```python
from build123d import *

# Parameters (mm, degrees)
CYLINDER084_R     = 2
CYLINDER084_DEPTH = 10
CYLINDER083_R     = 3.25
CYLINDER083_DEPTH = 10
CYLINDER082_R     = 2
CYLINDER082_DEPTH = 10
BOX069_W          = 8.5
BOX069_H          = 22
BOX069_DEPTH      = 25
BOX068_W          = 8
BOX068_H          = 22
BOX068_DEPTH      = 25


with BuildPart() as cylinder084:
    # Cylinder084 → Cylinder084 (new body)
    with BuildSketch(Plane(origin=(335, 287, 0), x_dir=(1, 0, 0), z_dir=(0, 0, 1))):
        Circle(CYLINDER084_R)
    extrude(amount=CYLINDER084_DEPTH)


with BuildPart() as cylinder083:
    # Cylinder083 → Cylinder083 (new body)
    with BuildSketch(Plane(origin=(335, 305, 17), x_dir=(1, 0, 0), z_dir=(0, -1, 0))):
        Circle(CYLINDER083_R)
    extrude(amount=CYLINDER083_DEPTH)


with BuildPart() as fusion049:
    # Cylinder082 → Cylinder082 (new body)
    with BuildSketch(Plane(origin=(335, 294, 0), x_dir=(1, 0, 0), z_dir=(0, 0, 1))):
        Circle(CYLINDER082_R)
    extrude(amount=CYLINDER082_DEPTH)

    # Fusion049: union Cylinder083
    add(cylinder083.part)


with BuildPart() as cube020:
    # Box069 → Box069 (new body)
    with BuildSketch(Plane(origin=(331, 278, 9), x_dir=(1, 0, 0), z_dir=(0, 0, 1))):
        with Locations((4.25, 11)):
            Rectangle(BOX069_W, BOX069_H)
    extrude(amount=BOX069_DEPTH)


with BuildPart() as antennaholder:
    # Box068 → Box068 (new body)
    with BuildSketch(Plane(origin=(331, 283, 0), x_dir=(1, 0, 0), z_dir=(0, 0, 1))):
        with Locations((4, 11)):
            Rectangle(BOX068_W, BOX068_H)
    extrude(amount=BOX068_DEPTH)

    # Cut061: cut Cube020
    add(cube020.part, mode=Mode.SUBTRACT)

    # Cut062: cut Fusion049
    add(fusion049.part, mode=Mode.SUBTRACT)

    # Cut063: cut Cylinder084
    add(cylinder084.part, mode=Mode.SUBTRACT)


solid = antennaholder.part
```
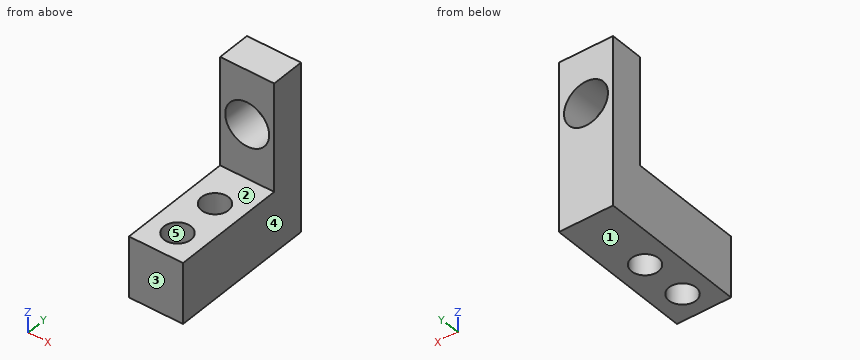
The listing builds one solid part. Answer for the finished solid, in the listing's coordinates (mm). Face numbers are marked on the shaded views. A direction names the side the tool comes from. Coordinates: 2 decimals unless noted, no trailing zeros. Loops run counter-clockwise (first coordinate to the right, second up) from the corner with the lowest first, then second, coordinate; pieces in that order, holes last. Notation, with made-up numbers: (-29, 2) - (-16, 2) arc R10 cw to (-16, 13) - close; hole circle Ø9 at (-15.5, 82). An arc over 180 degrees is marked (long way). Use a Markdown table: item, result. Add a question column.
1) The part is cut by section D-D, the plane x = 332.5. Give the vertices of the cut face in (y, z).
2) Given pin 1 (1 mm diameter, centred on x = 336.5, y = 287.5, fed in from +Z), flat-ended and moving along its own axis, determine where the tip first touches the part or whether it passes through.
3) The part is cut by section B-B, the plane x = 335. Give the vertices of the cut face in (y, z).
4) For the marked faces 1 and 2, determine the directions among +Z, -Z, +X, -X, +Y, -Y from which every point of the face is accessible in a straight line to the end or side of a thin tool.
5) The part is cut by section A-A, the plane y = 287. Give the vertices of the cut face in (x, z).
6) The mould has two halves that part along Y. Classify the marked faces 3, 4 and 5: released by +Y, released by -Y, zero draft, split by the parting line, or undercut.
7) Find the intervals of material crossed by line 1 (X direction, y = 303.35, z = 17); line 2 (Y direction, x = 333.5, z = 1); line 3 (Z direction, x = 335, y = 302.25), in increasing order.
8) The part is cut by section C-C, the plane y = 301.25. Give the vertices of the cut face in (x, z), and give its area (3 significant figures).
Here are the results:
| question | item | result |
|---|---|---|
| 1 | outline | (283, 0) - (305, 0) - (305, 14.92) - (300, 14.92) - (300, 9) - (283, 9) - close; (300, 19.08) - (305, 19.08) - (305, 25) - (300, 25) - close |
| 2 | pin 1 | stops at z = 9 |
| 3 | outline | (283, 0) - (285, 0) - (285, 9) - (283, 9) - close; (289, 0) - (292, 0) - (292, 9) - (289, 9) - close; (296, 0) - (305, 0) - (305, 13.75) - (300, 13.75) - (300, 9) - (296, 9) - close; (300, 20.25) - (305, 20.25) - (305, 25) - (300, 25) - close |
| 4 | face 1 | -Z, +X, -X, +Y, -Y |
| 4 | face 2 | +Z, +X, -X, -Y |
| 5 | outline | (331, 0) - (333, 0) - (333, 9) - (331, 9) - close; (337, 0) - (339, 0) - (339, 9) - (337, 9) - close |
| 6 | face 3 | released by -Y |
| 6 | face 4 | zero draft |
| 6 | face 5 | undercut |
| 7 | line 1 | x = 331 to 331.75, 338.25 to 339 |
| 7 | line 2 | y = 283 to 285.68, 288.32 to 292.68, 295.32 to 305 |
| 7 | line 3 | z = 0 to 13.75, 20.25 to 25 |
| 8 | outline | (331, 0) - (339, 0) - (339, 25) - (331, 25) - close; hole circle Ø6.5 at (335, 17) |
| 8 | area | 167 mm^2 |
